Source: CAD feature listing. Evaluate the final solid. Frame: model axes, mm. Give positions to 0.01 mm unless a question says otherwise; leave off trailing zeros. Order: outer loops, then holes, each group sorted by start corner. A loop starts at its lowest first (then second) coordinate and runs counter-clockwise, first axis right, second up. Notation, with made-up numbers: (-8, 25.25) - (21, 25.25) arc R10 cw to (21, 33.25) - close; hole circle Ø6 at (-16.75, 39). An arc over 180 degrees is marked (long way). Answer as CSV lines item,"result".
```python
from build123d import *

# Parameters (mm, degrees)
F0_W     = 228.6
F0_H     = 152.4
F1_DEPTH = 2.286
F2_R     = 1.6256
F3_DEPTH = 2.287
F4_SIZE  = 22.225


with BuildPart() as f1:
    # F0 (on Top) → F1 (new body)
    with BuildSketch(Plane.XY):
        Rectangle(F0_W, F0_H)
    extrude(amount=-F1_DEPTH)

    # F2 (on face) → F3 (cut, through all)
    with BuildSketch(Plane.XY):
        with Locations((-76.2, 0)):
            Circle(F2_R)
        with Locations((76.2, 0)):
            Circle(F2_R)
    extrude(amount=-F3_DEPTH, mode=Mode.SUBTRACT)

    # F4
    f4_edges = [f1.edges().sort_by_distance(p)[0] for p in [
        (-114.3, 76.2, -1.143),
        (114.3, 76.2, -1.143),
        (-114.3, -76.2, -1.143),
        (114.3, -76.2, -1.143),
    ]]
    chamfer(f4_edges, length=F4_SIZE)


solid = f1.part
```
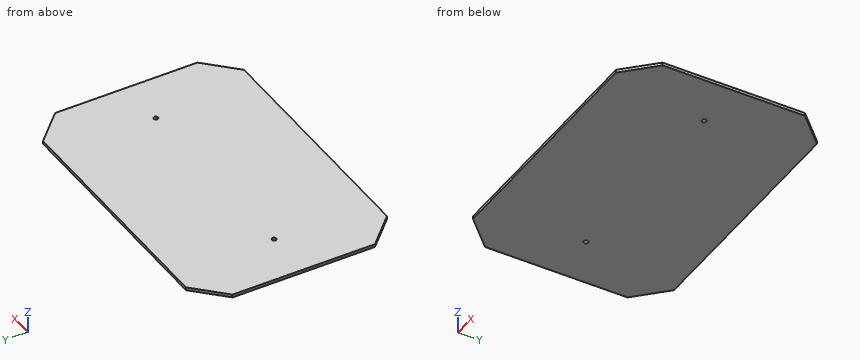
(1) Contact query for a flat-ended pin moving along its axis: pin 1 (4 mm diameter, centred on x = 65.5, y = -17, fed in from +Z). Output: stop coordinate, or through.
Completed:
pin 1,"z = 0"
(2) Cut plane A-A (z = -0.85). Return loops of the section in (x, y) (3 decimals), then the cut area to 3 significant figures.
Completed:
outline,"(-114.3, -53.975) - (-92.075, -76.2) - (92.075, -76.2) - (114.3, -53.975) - (114.3, 53.975) - (92.075, 76.2) - (-92.075, 76.2) - (-114.3, 53.975) - close; hole circle Ø3.251 at (-76.2, 0); hole circle Ø3.251 at (76.2, 0)"
area,"33,800 mm²"
(3) Cut plane C-C (x = 98.5). Return loops of the section in (y, z) (3 decimals).
Completed:
outline,"(-69.775, -2.286) - (69.775, -2.286) - (69.775, 0) - (-69.775, 0) - close"
(4) Cut plane B-B (y = -58). Return loops of the section in (x, z) (3 decimals).
Completed:
outline,"(-110.275, -2.286) - (110.275, -2.286) - (110.275, 0) - (-110.275, 0) - close"
(5) Ray query, line 1 (Y direction, x = -76.2, z = -1.7); line 2 (Y direction, x = -104, z = -1.7) (3 decimals). Return the intervals inside material, ascending. Write a range as from..to.
Completed:
line 1,"-76.2..-1.63, 1.63..76.2"
line 2,"-64.275..64.275"
